Geometry: final body of the model. Coordinates: model frame, mm. A direction names the side the tool comes from. Give positions to 0.01 mm unless a question says otherwise; leave off trailing zeros. Loops run counter-clockwise (first coordinate to the right, second up) from the corner with the lowest first, then second, coordinate; pieces in that order, holes last.
1. Draft query along Y for faces 5 (the face through (-0.99, 5.59, 6.85)), 6 (the face through (1.97, -6.31, -0.66)), 7 (the face through (1.01, -0.91, 9.25)), 8 (the face through (0.986, -2.766, -46.049)). Return one class per face: +Y half, -Y half, draft (parallel to the pull), parting line (faces both ways), or undercut.
2. Section D-D, the plane x = 2.8. Output: boundary loops of the cut face in (y, z).
3. Material intervals for line 1 along Y through (x, z) = (-1.2, 7.5); line 2 along X through (y, z) = (-3.75, -32.5); line 3 along Y through (x, z) = (1.5, -22), sorted ascending.
4. Section C-C, the plane y = 7.5. Output: boundary loops of the cut face in (x, z).
5. Section B-B, the plane x = -0.7. Output: boundary loops of the cut face in (y, z).
6. Section A-A, the plane z = -35. Output: boundary loops of the cut face in (x, y).
7. Access query for faces 1 (the face through (1.014, 0.216, -40.421)), 2 (the face through (2.99, -5.32, -0.53)), 3 (the face through (-2, 4, 8)), 4 (the face through (1, -6, -26)). Directions: +Z, -Z, +X, -X, +Y, -Y. A direction counts if a zero-diameter tool reaches every point of the face in a straight line with its end or side. Return the directions, or none.
8. First-contact query: P1, Ø11, axis at y = 0, z = -15, coming from the +X side; P2, Ø1, axis at x = 0.5, z = -23, coming from the -Y side; P3, Ø8, axis at y = -11, z = -38, coming from the +X side; P4, Ø0.6, axis at x = 1, z = -22, coming from the +Y side. Flat tips, straight axial feed; report the tip coordinate or a pass-through.
from build123d import *

# Parameters (mm, degrees)
EXTRUDE_1_DEPTH          = 2
EXTRUDE_START            = 2
SKETCH_1_4_R             = 3
EXTRUDE_2_DEPTH          = 2
CUT_EXTRUDE_1_DEPTH      = 51.160727735
CUT_EXTRUDE_1_DEPTH_BACK = 51.160727735
SKETCH_1_3_R             = 2
FILLET_1_R               = 3
SKETCH_2_R               = 2
EXTRUDE_3_DEPTH          = 2
SKETCH_2_3_R             = 1.8
EXTRUDE_4_DEPTH          = 2


with BuildPart() as part:
    # 草图1 → 凸台-拉伸1 (new body)
    with BuildSketch(Plane(origin=(0, 0, 0), x_dir=(0, 0, -1), z_dir=(1, 0, 0))):
        with BuildLine():
            Line((40.737143614, 0), (0, 0))
            Line((0, 0), (2.48051592, -3.542543867))
            ThreePointArc((2.48051592, -3.542543867), (4.165783411, -4.487079684), (5.367176995, -6))
            Line((5.367176995, -6), (44.201245229, -6))
            ThreePointArc((44.201245229, -6), (40.737143614, -4), (40.737143614, 0))
        make_face()
        with BuildLine():
            Line((2.48051592, -3.542543867), (0, 0))
            Line((0, 0), (-2.681672007, 3.829824531))
            ThreePointArc((-2.681672007, 3.829824531), (-4.811127311, -0.102785303), (-9.234888361, -0.758786959))
            Line((-9.234888361, -0.758786959), (-4.072700434, -8.131155358))
            ThreePointArc((-4.072700434, -8.131155358), (-1.94324513, -4.198545524), (2.48051592, -3.542543867))
        make_face()
        with BuildLine():
            ThreePointArc((48.201245229, -2), (45.23652141, 1.863703305), (40.737143614, 0))
            Line((40.737143614, 0), (44.201245229, 0))
            ThreePointArc((44.201245229, 0), (45.615458792, -0.585786438), (46.201245229, -2))
            ThreePointArc((46.201245229, -2), (45.615458792, -3.414213562), (44.201245229, -4))
            Line((44.201245229, -4), (44.201245229, -6))
            ThreePointArc((44.201245229, -6), (47.029672354, -4.828427125), (48.201245229, -2))
        make_face()
        with BuildLine():
            Line((44.201245229, 0), (40.737143614, 0))
            ThreePointArc((40.737143614, 0), (40.737143614, -4), (44.201245229, -6))
            Line((44.201245229, -6), (44.201245229, -4))
            ThreePointArc((44.201245229, -4), (42.201245229, -2), (44.201245229, 0))
        make_face()
        with BuildLine():
            ThreePointArc((5.367176995, -6), (4.165783411, -4.487079684), (2.48051592, -3.542543867))
            Line((2.48051592, -3.542543867), (4.201245229, -6))
            Line((4.201245229, -6), (5.367176995, -6))
        make_face()
        with BuildLine():
            Line((4.201245229, -6), (2.48051592, -3.542543867))
            ThreePointArc((2.48051592, -3.542543867), (-1.94324513, -4.198545524), (-4.072700434, -8.131155358))
            Line((-4.072700434, -8.131155358), (-2.351971125, -10.588611491))
            Line((-2.351971125, -10.588611491), (-1.532819081, -10.015035054))
            ThreePointArc((-1.532819081, -10.015035054), (-0.796092257, -5.836849613), (3.382093185, -6.573576436))
            Line((3.382093185, -6.573576436), (4.201245229, -6))
        make_face()
        with BuildLine():
            ThreePointArc((-9.234888361, -0.758786959), (-4.811127311, -0.102785303), (-2.681672007, 3.829824531))
            Line((-2.681672007, 3.829824531), (-4.402401316, 6.287280664))
            Line((-4.402401316, 6.287280664), (-6.040705405, 5.140127792))
            ThreePointArc((-6.040705405, 5.140127792), (-5.771575592, 4.594386518), (-5.679009493, 3.992974919))
            ThreePointArc((-5.679009493, 3.992974919), (-7.077597894, 2.085541017), (-9.317313582, 2.845822046))
            Line((-9.317313582, 2.845822046), (-10.95561767, 1.698669174))
            Line((-10.95561767, 1.698669174), (-9.234888361, -0.758786959))
        make_face()
        with BuildLine():
            Line((-4.402401316, 6.287280664), (-2.681672007, 3.829824531))
            ThreePointArc((-2.681672007, 3.829824531), (-2.679675166, 3.911388863), (-2.679009493, 3.992974919))
            ThreePointArc((-2.679009493, 3.992974919), (-10.613341245, 8.041394014), (-9.234888361, -0.758786959))
            Line((-9.234888361, -0.758786959), (-10.95561767, 1.698669174))
            Line((-10.95561767, 1.698669174), (-9.317313582, 2.845822046))
            ThreePointArc((-9.317313582, 2.845822046), (-8.826162366, 5.631279008), (-6.040705405, 5.140127792))
            Line((-6.040705405, 5.140127792), (-4.402401316, 6.287280664))
        make_face()
        with BuildLine():
            ThreePointArc((46.201245229, -2), (45.615458792, -0.585786438), (44.201245229, 0))
            Line((44.201245229, 0), (44.201245229, -4))
            ThreePointArc((44.201245229, -4), (45.615458792, -3.414213562), (46.201245229, -2))
        make_face()
        with BuildLine():
            Line((44.201245229, -4), (44.201245229, 0))
            ThreePointArc((44.201245229, 0), (42.201245229, -2), (44.201245229, -4))
        make_face()
        with BuildLine():
            Line((5.367176995, -6), (4.201245229, -6))
            Line((4.201245229, -6), (3.382093185, -6.573576436))
            ThreePointArc((3.382093185, -6.573576436), (3.785787904, -7.392188347), (3.924637052, -8.294305745))
            ThreePointArc((3.924637052, -8.294305745), (1.826754451, -11.155456598), (-1.532819081, -10.015035054))
            Line((-1.532819081, -10.015035054), (-2.351971125, -10.588611491))
            Line((-2.351971125, -10.588611491), (-4.072700434, -8.131155358))
            ThreePointArc((-4.072700434, -8.131155358), (0.843050996, -13.293640073), (5.924637052, -8.294305745))
            ThreePointArc((5.924637052, -8.294305745), (5.783273678, -7.113776143), (5.367176995, -6))
        make_face()
        with BuildLine():
            ThreePointArc((3.924637052, -8.294305745), (3.785787904, -7.392188347), (3.382093185, -6.573576436))
            Line((3.382093185, -6.573576436), (2.562941141, -7.147152873))
            ThreePointArc((2.562941141, -7.147152873), (2.832070954, -7.692894146), (2.924637052, -8.294305745))
            ThreePointArc((2.924637052, -8.294305745), (1.526048651, -10.201739647), (-0.713667036, -9.441458618))
            Line((-0.713667036, -9.441458618), (-1.532819081, -10.015035054))
            ThreePointArc((-1.532819081, -10.015035054), (1.826754451, -11.155456598), (3.924637052, -8.294305745))
        make_face()
        with BuildLine():
            Line((2.562941141, -7.147152873), (3.382093185, -6.573576436))
            ThreePointArc((3.382093185, -6.573576436), (-0.796092257, -5.836849613), (-1.532819081, -10.015035054))
            Line((-1.532819081, -10.015035054), (-0.713667036, -9.441458618))
            ThreePointArc((-0.713667036, -9.441458618), (-0.222515821, -6.656001657), (2.562941141, -7.147152873))
        make_face()
        with BuildLine():
            ThreePointArc((-5.679009493, 3.992974919), (-5.771575592, 4.594386518), (-6.040705405, 5.140127792))
            Line((-6.040705405, 5.140127792), (-9.317313582, 2.845822046))
            ThreePointArc((-9.317313582, 2.845822046), (-7.077597894, 2.085541017), (-5.679009493, 3.992974919))
        make_face()
        with BuildLine():
            Line((-9.317313582, 2.845822046), (-6.040705405, 5.140127792))
            ThreePointArc((-6.040705405, 5.140127792), (-8.826162366, 5.631279008), (-9.317313582, 2.845822046))
        make_face()
        with BuildLine():
            ThreePointArc((2.924637052, -8.294305745), (2.832070954, -7.692894146), (2.562941141, -7.147152873))
            Line((2.562941141, -7.147152873), (-0.713667036, -9.441458618))
            ThreePointArc((-0.713667036, -9.441458618), (1.526048651, -10.201739647), (2.924637052, -8.294305745))
        make_face()
        with BuildLine():
            Line((-0.713667036, -9.441458618), (2.562941141, -7.147152873))
            ThreePointArc((2.562941141, -7.147152873), (-0.222515821, -6.656001657), (-0.713667036, -9.441458618))
        make_face()
    extrude(amount=EXTRUDE_1_DEPTH)

    # 草图1<4> → 凸台-拉伸2 (add)
    with BuildSketch(Plane(origin=(0, 0, 0), x_dir=(0, 0, -1), z_dir=(1, 0, 0)).offset(EXTRUDE_START)):
        with Locations((0.924637052, -8.294305745)):
            Circle(SKETCH_1_4_R)
    extrude(amount=EXTRUDE_2_DEPTH)

    # 草图1<3> → 切除-拉伸1 (cut, two sides: drawn at the far end of the back side and taken through both)
    with BuildSketch(Plane(origin=(0, 0, 0), x_dir=(0, 0, -1), z_dir=(1, 0, 0)).offset(-CUT_EXTRUDE_1_DEPTH_BACK)):
        with Locations((-7.679009493, 3.992974919)):
            Circle(SKETCH_1_3_R)
        with Locations((44.201245229, -2)):
            Circle(SKETCH_1_3_R)
        with Locations((0.924637052, -8.294305745)):
            Circle(SKETCH_1_3_R)
    extrude(amount=CUT_EXTRUDE_1_DEPTH + CUT_EXTRUDE_1_DEPTH_BACK, mode=Mode.SUBTRACT)

    # 圆角1
    fillet_1_edges = [part.edges().sort_by_distance(p)[0] for p in [
        (1, -6, -5.367176995),
        (1, 0, 0),
        (1, 0, -40.737143614),
        (1, -0.758786959, 9.234888361),
        (1, -8.131155358, 4.072700434),
    ]]
    fillet(fillet_1_edges, radius=FILLET_1_R)

    # 草图2 → 凸台-拉伸3 (add)
    with BuildSketch(Plane.ZY):
        with Locations((7.679009493, 3.992974919)):
            Circle(SKETCH_2_R)
    extrude(amount=-EXTRUDE_3_DEPTH)

    # 草图2<3> → 凸台-拉伸4 (add)
    with BuildSketch(Plane.ZY):
        with Locations(Location((7.679009493, 3.992974919, 0), (0, 0, 180))):
            Circle(SKETCH_2_3_R)
    extrude(amount=EXTRUDE_4_DEPTH)


solid = part.part
Answers below:
1. face 5: parting line
1. face 6: undercut
1. face 7: -Y half
1. face 8: undercut
2. outline: circle Ø6 at (-8.29, -0.92); hole circle Ø4 at (-8.29, -0.92)
3. line 1: y = 2.2 to 5.78
3. line 2: x = 0 to 2
3. line 3: y = -6 to 0
4. outline: (0, 4.12) - (2, 4.12) - (2, 11.24) - (0, 11.24) - close
5. outline: circle Ø3.6 at (3.99, 7.68)
6. outline: (0, -6) - (2, -6) - (2, 0) - (0, 0) - close
7. face 1: +X, -X, +Y
7. face 2: +X
7. face 3: +Z, -Z, -X, +Y, -Y
7. face 4: -Z, +X, -X, -Y
8. P1: stops at x = 2
8. P2: stops at y = -6
8. P3: passes through
8. P4: stops at y = 0
